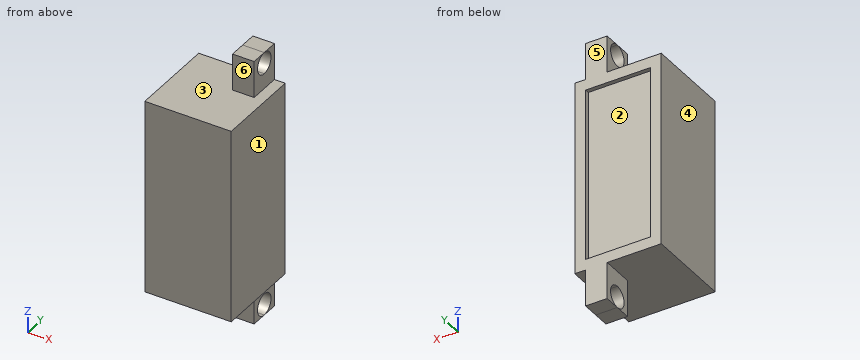
Autodesk Inventor part; units mm, degrees
ref_plane "YZ Plane" through (0, 0, 0) normal (1, 0, 0) x (0, 1, 0)
ref_plane "XZ Plane" through (0, 0, 0) normal (0, 1, 0) x (-1, 0, 0)
ref_plane "XY Plane" through (0, 0, 0) normal (0, 0, 1) x (1, 0, 0)
sketch "Sketch1" plane through (0, 0, 0) normal (0, 1, 0) x (-1, 0, 0)
  line L0 (20, 45) -> (-20, 45)
  line L1 (-20, 45) -> (-20, -45)
  line L2 (-20, -45) -> (20, -45)
  line L3 (20, -45) -> (20, 45)
  point P0 (0, 0)
  point P1 (20, 0)
  point P2 (0, -45)
  dimension "d0" = 40
  dimension "d1" = 90
extrude "Extrusion1" add sketch "Sketch1" along normal blind 40
sketch "Sketch2" plane through (-20, 0, 45) normal (0, 0, 1) x (1, 0, 0)
  line L0 (0, 40) -> (40, 40)
  line L1 (35, 40) -> (25, 40)
  line L2 (25, 40) -> (25, 25)
  line L3 (25, 25) -> (35, 25)
  line L4 (35, 25) -> (35, 40)
  line L5 (40, 0) -> (40, 40)
  point P0 (20, 0)
  dimension "d4" = 5
  dimension "d5" = 10
  dimension "d6" = 15
extrude "Extrusion2" add sketch "Sketch2" along normal blind 17
sketch "Sketch3" plane through (15, 25, 45) normal (1, 0, 0) x (0, 0, -1)
  circle A0 centre (-12, 7.5) radius 5
  line L0 (-17, 0) -> (-17, 15)
  line L1 (0, 15) -> (-17, 15)
  point P0 (45, -25)
  dimension "d9" = 10
  dimension "d10" = 5
  dimension "d11" = 7.5
extrude "Extrusion3" cut sketch "Sketch3" against normal blind 17
mirror "Mirror3" about plane through (0, 0, 0) normal (0, 0, 1) of "Extrusion2", "Extrusion3"
sketch "Sketch4" plane through (0, 40, 0) normal (0, 1, 0) x (1, 0, 0)
  line L0 (-15, -40) -> (15, -40)
  line L1 (15, -40) -> (15, 40)
  line L2 (15, 40) -> (-15, 40)
  line L3 (-15, 40) -> (-15, -40)
  point P0 (0, 0)
  point P1 (-15, 0)
  point P2 (0, -40)
  dimension "d14" = 80
  dimension "d15" = 30
extrude "Extrusion4" cut sketch "Sketch4" against normal blind 2
properties part number "speaker"
The model under review builds one solid part; all positions refer to its coordinate system, in mm. Face numbers are marked on the shaded views. A direction names the side the tool comes from. Round coordinates to 2 decimals unless told otherwise and drop trailing zeros. Loops run counter-clockwise (first coordinate to the right, second up) from the corner with the lowest first, then second, coordinate; pieces in that order, holes last. Notation, with made-up numbers: (22, -13) -> (40, -13) arc R32 ccw to (40, 20) -> close; hole circle Ø3 at (43, 52). An arc over 180 degrees is marked (long way). Answer in a Markdown table with one row per item.
1) Consider section D-D, the plane x = -2. Write out the cut boundary in (y, z).
Taken from the geometry:
| item | result |
|---|---|
| outline | (0, -45) -> (40, -45) -> (40, -40) -> (38, -40) -> (38, 40) -> (40, 40) -> (40, 45) -> (0, 45) -> close |
2) Draft analysis for pull direction X (two halves, no side actions). For the marked faces 1, 2, 3 and 4, state which applies: pulls with the +X half, pulls with the -X half, needs draft (parallel to the pull), parting line crosses it, or undercut.
Taken from the geometry:
| item | result |
|---|---|
| face 1 | pulls with the +X half |
| face 2 | undercut |
| face 3 | needs draft |
| face 4 | pulls with the -X half |
3) Consider section B-B, the plane y = 35.5. Write out the cut boundary in (x, z), plus the area to 3 significant figures.
Taken from the geometry:
| item | result |
|---|---|
| outline | (-20, -45) -> (5, -45) -> (5, -53) -> (15, -53) -> (15, -45) -> (20, -45) -> (20, 45) -> (15, 45) -> (15, 53) -> (5, 53) -> (5, 45) -> (-20, 45) -> close; (5, -62) -> (15, -62) -> (15, -61) -> (5, -61) -> close; (5, 61) -> (15, 61) -> (15, 62) -> (5, 62) -> close |
| area | 3,780 mm² |
4) For pin 1 Ø9 at (x, z) = (5.5, -13) entering from +Y; pin 2 Ø16.5 at (y, z) = (33, -53.5) entering from -X; pin 3 Ø2 at (x, y) = (-8.5, 5.5) entering from -Z, all flat-tipped, find the tip position at first contact; note any pin that passes through.
Taken from the geometry:
| item | result |
|---|---|
| pin 1 | stops at y = 38 |
| pin 2 | stops at x = 5 |
| pin 3 | stops at z = -45 |
5) Tool access review of the marked faces 5 and 6: name each direction out of +Z, -Z, +X, -X, +Y, -Y from which nothing blocks a thin tool from reaching the whole face with its end or side.
Taken from the geometry:
| item | result |
|---|---|
| face 5 | +Z, -Z, +X, -X, +Y |
| face 6 | +Z, +X, -X, -Y |
6) Wall thickness on line 1 along Z through (x, y) = (14, 37); line 2 along Z through (x, y) = (14.5, 36); line 3 along Y through (x, z) = (11, 25.5): over which ranges is each line inside the solid? List them lowest first.
Taken from the geometry:
| item | result |
|---|---|
| line 1 | z = -62 to -59.18, -54.82 to 54.82, 59.18 to 62 |
| line 2 | z = -62 to -60.57, -53.43 to 53.43, 60.57 to 62 |
| line 3 | y = 0 to 38 |
7) Consider section A-A, the plane z = -57. Write out the cut boundary in (x, y).
Taken from the geometry:
| item | result |
|---|---|
| outline | (5, 25) -> (15, 25) -> (15, 27.5) -> (5, 27.5) -> close; (5, 37.5) -> (15, 37.5) -> (15, 40) -> (5, 40) -> close |
